from build123d import *

# Parameters (mm, degrees)
SKETCH_1_W          = 65
SKETCH_1_H          = 25
EXTRUDE_1_DEPTH     = 4
SKETCH_2_W          = 15
SKETCH_2_H          = 25
EXTRUDE_2_DEPTH     = 13
SKETCH_3_R          = 2.6
SKETCH_3_R_2        = 4
CUT_EXTRUDE_1_DEPTH = 39.74919354
SKETCH_5_W          = 15
SKETCH_5_H          = 4
EXTRUDE_3_DEPTH     = 6
SKETCH_6_R          = 1.25
CUT_EXTRUDE_3_DEPTH = 40.59166579
FILLET_2_R          = 3
CUT_EXTRUDE_4_DEPTH = 49.023431781
SKETCH_9_W          = 15
SKETCH_9_H          = 4
CUT_EXTRUDE_5_DEPTH = 42.403502267


with BuildPart() as part:
    # 草图1 → 凸台-拉伸1 (new body)
    with BuildSketch(Plane(origin=(0, 0, 0), x_dir=(1, 0, 0), z_dir=(0, 1, 0))):
        Rectangle(SKETCH_1_W, SKETCH_1_H)
    extrude(amount=EXTRUDE_1_DEPTH)

    # 草图2 → 凸台-拉伸2 (add)
    with BuildSketch(Plane(origin=(0, 4, 0), x_dir=(1, 0, 0), z_dir=(0, 1, 0))):
        Rectangle(SKETCH_2_W, SKETCH_2_H)
    extrude(amount=EXTRUDE_2_DEPTH)

    # 草图3 → 切除-拉伸1 (cut, through all)
    with BuildSketch(Plane.XZ):
        with Locations(Location((0, -7.5, 0), (0, 0, 270))):
            Circle(SKETCH_3_R)
        with Locations(Location((0, 7.5, 0), (0, 0, 90))):
            Circle(SKETCH_3_R)
        with Locations(Location((-22, 0, 0), (0, 0, 270))):
            Circle(SKETCH_3_R_2)
        with Locations(Location((22, 0, 0), (0, 0, 90))):
            Circle(SKETCH_3_R_2)
    extrude(amount=-CUT_EXTRUDE_1_DEPTH, mode=Mode.SUBTRACT)

    # 草图5 → 凸台-拉伸3 (add)
    with BuildSketch(Plane.XY.offset(12.5)):
        with Locations((0, 6)):
            Rectangle(SKETCH_5_W, SKETCH_5_H)
    extrude_3 = extrude(amount=EXTRUDE_3_DEPTH)

    # 草图6 → 切除-拉伸3 (cut, through all)
    with BuildSketch(Plane.XZ.offset(-4)):
        with Locations(Location((-4.5, 15.5, 0), (0, 0, 270))):
            Circle(SKETCH_6_R)
        with Locations(Location((4.5, 15.5, 0), (0, 0, 270))):
            Circle(SKETCH_6_R)
    cut_extrude_3 = extrude(amount=-CUT_EXTRUDE_3_DEPTH, mode=Mode.SUBTRACT)

    # 镜向2: 凸台-拉伸3, 切除-拉伸3 across plane
    add(extrude_3.mirror(Plane.XY))
    add(cut_extrude_3.mirror(Plane.XY), mode=Mode.SUBTRACT)

    # 圆角2
    fillet_2_edges = [part.edges().sort_by_distance(p)[0] for p in [
        (-7.5, 6, 18.5),
        (7.5, 6, 18.5),
        (-7.5, 6, -18.5),
        (7.5, 6, -18.5),
    ]]
    fillet(fillet_2_edges, radius=FILLET_2_R)

    # 草图7 → 切除-拉伸4 (cut, through all)
    with BuildSketch(Plane(origin=(0, 0, -12.5), x_dir=(-1, 0, 0), z_dir=(0, 0, -1))):
        Polygon((32.5, 4), (7.5, 4), (-7.5, 4), (-32.5, 4), (-32.5, 0), (32.5, 0), align=None)
    extrude(amount=-CUT_EXTRUDE_4_DEPTH, mode=Mode.SUBTRACT)

    # 草图9 → 切除-拉伸5 (cut, through all)
    with BuildSketch(Plane.XY.offset(18.5)):
        with Locations((0, 6)):
            Rectangle(SKETCH_9_W, SKETCH_9_H)
    extrude(amount=-CUT_EXTRUDE_5_DEPTH, mode=Mode.SUBTRACT)


solid = part.part
Geometry: final body of the model. Coordinates: model frame, mm. Coordinates: 2 decimals unless noted, no trailing zeros. Order: outer loops, then holes, each group sorted by start corner. A loop starts at its lowest first (then second) coordinate and runs counter-clockwise, first axis right, second up.
1) Ray query, probe 1 along X at (y, z) = (11.5, 7.5); probe 2 along Z at (x, y) = (0.75, 16); probe 3 along Z at (x, y) = (1.5, 13.25). Return the intervals inside material, ascending.
Result sheet:
probe 1: x = -7.5 to -2.6, 2.6 to 7.5
probe 2: z = -12.5 to -9.99, -5.01 to 5.01, 9.99 to 12.5
probe 3: z = -12.5 to -9.62, -5.38 to 5.38, 9.62 to 12.5
2) Section C-C (y = 13). Return loops of the section in (x, z).
Result sheet:
outline: (-7.5, -12.5) - (7.5, -12.5) - (7.5, 12.5) - (-7.5, 12.5) - close; hole circle Ø5.2 at (0, -7.5); hole circle Ø5.2 at (0, 7.5)
3) Section B-B (x = 0). Return loops of the section in (y, z).
Result sheet:
outline: (8, -12.5) - (17, -12.5) - (17, -10.1) - (8, -10.1) - close; (8, -4.9) - (17, -4.9) - (17, 4.9) - (8, 4.9) - close; (8, 10.1) - (17, 10.1) - (17, 12.5) - (8, 12.5) - close
4) Section D-D (z = 6). Return loops of the section in (x, y), then the cut area to 3 significant figures.
Result sheet:
outline: (-7.5, 8) - (-2.12, 8) - (-2.12, 17) - (-7.5, 17) - close; (2.12, 8) - (7.5, 8) - (7.5, 17) - (2.12, 17) - close
area: 96.8 mm2
5) First-contact query: P1, Ø8.5, axis at x = 0, z = 7.5, coming from the -Y side. Flat tip, straight axial feed; report the tip coordinate or a pass-through.
Result sheet:
P1: stops at y = 8
6) Section A-A (z = -7.5). Return loops of the section in (x, y).
Result sheet:
outline: (-7.5, 8) - (-2.6, 8) - (-2.6, 17) - (-7.5, 17) - close; (2.6, 8) - (7.5, 8) - (7.5, 17) - (2.6, 17) - close
7) Draft query along X for faces 1 (the flat face through (-7.5, 12, 0)), 2 (the flat face through (7.5, 12, 0)), 3 (the cylindrical face through (-0.78, 12.44, 9.98)), 4 (the cylindrical face through (0.78, 12.44, -9.98)). Return one class per face: released by +X, released by -X, zero draft, split by the parting line, or undercut.
Result sheet:
face 1: released by -X
face 2: released by +X
face 3: undercut
face 4: undercut
